```python
from build123d import *

# Parameters (mm, degrees)
RETAINER_PLATE_2MM_START         = -2
RETAINER_PLATE_2MM_DEPTH         = 2
RETAINER_PLATE_2MM_ROOT_START    = -2
SKETCH_2_R                       = 10
RETAINER_PLATE_2MM_ROOT_DEPTH    = 2
RETAINER_PLATE_2MM_TIP_START     = -2
SKETCH_3_R                       = 10
RETAINER_PLATE_2MM_TIP_DEPTH     = 2
HORN_CONTACT_PAD_0P15_DEPTH      = 0.15
SKETCH_5_R                       = 3.8
HORN_CONTACT_PAD_0P15_ROOT_DEPTH = 0.15
SKETCH_6_R                       = 1.35
HORN_CONTACT_PAD_0P15_TIP_DEPTH  = 0.15
BOSS_CLEARANCE_8_START           = -2.1
SKETCH_7_R                       = 4
BOSS_CLEARANCE_8_DEPTH           = 2.5
M2_CLEARANCE_2P5_PITCH14_START   = -2.1
SKETCH_8_R                       = 1.25
M2_CLEARANCE_2P5_PITCH14_DEPTH   = 2.5


with BuildPart() as part:
    # 草图1 → Retainer_plate_2mm (new body)
    with BuildSketch(Plane.XY.offset(RETAINER_PLATE_2MM_START)):
        Polygon((8.660254038, -5), (18.660254038, 12.320508076), (1.339745962, 22.320508076), (-8.660254038, 5), align=None)
    extrude(amount=RETAINER_PLATE_2MM_DEPTH)

    # 草图2 → Retainer_plate_2mm_root (add)
    with BuildSketch(Plane.XY.offset(RETAINER_PLATE_2MM_ROOT_START)):
        Circle(SKETCH_2_R)
    extrude(amount=RETAINER_PLATE_2MM_ROOT_DEPTH)

    # 草图3 → Retainer_plate_2mm_tip (add)
    with BuildSketch(Plane.XY.offset(RETAINER_PLATE_2MM_TIP_START)):
        with Locations((10, 17.320508076)):
            Circle(SKETCH_3_R)
    extrude(amount=RETAINER_PLATE_2MM_TIP_DEPTH)

    # 草图4 → Horn_contact_pad_0p15 (add)
    with BuildSketch(Plane.XY):
        Polygon((3.290896534, -1.9), (10.319134295, 15.173264889), (7.980865705, 16.523264889), (-3.290896534, 1.9), align=None)
    extrude(amount=HORN_CONTACT_PAD_0P15_DEPTH)

    # 草图5 → Horn_contact_pad_0p15_root (add)
    with BuildSketch(Plane.XY):
        Circle(SKETCH_5_R)
    extrude(amount=HORN_CONTACT_PAD_0P15_ROOT_DEPTH)

    # 草图6 → Horn_contact_pad_0p15_tip (add)
    with BuildSketch(Plane.XY):
        with Locations((9.15, 15.848264889)):
            Circle(SKETCH_6_R)
    extrude(amount=HORN_CONTACT_PAD_0P15_TIP_DEPTH)

    # 草图7 → Boss_clearance_8 (cut)
    with BuildSketch(Plane.XY.offset(BOSS_CLEARANCE_8_START)):
        with Locations(Location((0, 0, 0), (0, 0, 122.696435406))):
            Circle(SKETCH_7_R)
    extrude(amount=BOSS_CLEARANCE_8_DEPTH, mode=Mode.SUBTRACT)

    # 草图8 → M2_clearance_2p5_pitch14 (cut)
    with BuildSketch(Plane.XY.offset(M2_CLEARANCE_2P5_PITCH14_START)):
        with Locations((10.062177826, 3.42820323)):
            Circle(SKETCH_8_R)
        with Locations((-2.062177826, 10.42820323)):
            Circle(SKETCH_8_R)
    extrude(amount=M2_CLEARANCE_2P5_PITCH14_DEPTH, mode=Mode.SUBTRACT)


solid = part.part
```
Work out the finished part from the listing and answer in its coordinate system (mm). A direction names the side the tool comes from. Give positions to 0.01 mm unless a question says otherwise; leave off trailing zeros. Order: outer loops, then holes, each group sorted by start corner. A loop starts at its lowest first (then second) coordinate and runs counter-clockwise, first axis right, second up.
1. Section C-C, the plane z = -1.2 is taken. Determine the outline of the cut face in (x, y), and give its area (3 significant figures).
Result sheet:
outline: (-8.66, 5) arc R10 ccw to (8.66, -5) - (18.66, 12.32) arc R10 ccw to (1.34, 22.32) - close; hole circle Ø8 at (0, 0); hole circle Ø2.5 at (-2.06, 10.43); hole circle Ø2.5 at (10.06, 3.43)
area: 654 mm2
2. For faces 1 (the flat face through (8, 9, 0)), 2 (the flat face through (13.59, 3.54, -1.01)), determine the directions among +Z, -Z, +X, -X, +Y, -Y from which every point of the face is accessible in a straight line to the end or side of a thin tool.
Result sheet:
face 1: +Z
face 2: +Z, -Z, +X, -Y
3. Section A-A, the plane y = 10 is taken. Determine the outline of the cut face in (x, z).
Result sheet:
outline: (-5.77, -2) - (-3.24, -2) - (-3.24, 0) - (-5.77, 0) - close; (-0.89, -2) - (17.32, -2) - (17.32, 0) - (8.19, 0) - (8.19, 0.15) - (2.95, 0.15) - (2.95, 0) - (-0.89, 0) - close
4. Straight lines are drawn through the part: L1, parallel to Z at x = 6.75, y = -3.5; L2, parallel to X at y = 10, z = -1.8; L3, parallel to X at y = -2, z = -0.05. For each, find the intervals that lie inside material, in ascending order.
Result sheet:
L1: z = -2 to 0
L2: x = -5.77 to -3.24, -0.89 to 17.32
L3: x = -9.8 to -3.46, 3.46 to 10.39
5. The mould has two halves that part along Y. Classify faces 3 (the cylindrical face through (11.254, 3.804, -1.014)), 4 (the flat face through (5, 9, -2)), 5 (the cylindrical face through (-5.19, -8.55, -1.01)): released by +Y, released by -Y, zero draft, split by the parting line, or undercut.
Result sheet:
face 3: undercut
face 4: zero draft
face 5: split by the parting line
6. Section D-D, the plane y = -3.5 is taken. Determine the outline of the cut face in (x, z), and give its area (3 significant figures).
Result sheet:
outline: (-9.37, -2) - (-1.94, -2) - (-1.94, 0) - (-9.37, 0) - close; (1.94, -2) - (9.53, -2) - (9.53, 0) - (1.94, 0) - close
area: 30.0 mm2
7. Section B-B, the plane x = 0 is taken. Determine the outline of the cut face in (y, z).
Result sheet:
outline: (-10, -2) - (-4, -2) - (-4, 0) - (-10, 0) - close; (4, -2) - (20, -2) - (20, 0) - (6.17, 0) - (6.17, 0.15) - (4, 0.15) - close
8. Each of these flat-tipped pins is pushed along its axis until it touches: P1, Ø4, axis at x = -2, y = 9.5, coming from the -Z side; P2, Ø3, axis at x = 10.06, y = 3.43, coming from the +Z side. Where does it stop, or does it pass through?
Result sheet:
P1: stops at z = -2
P2: stops at z = 0
